For this review, take the finished solid that the model builds, in its own axes (mm). A direction names the side the tool comes from. Round coordinates to 2 decimals unless told otherwise and drop trailing zeros. Order: outer loops, then holes, each group sorted by start corner. A loop starts at its lowest first (then second) coordinate and runs counter-clockwise, first axis right, second up. Notation, with made-up numbers: (24.5, 24.5) - (74.5, 24.5) arc R30 ccw to (74.5, 46.5) - close; hole circle Ø11 at (89.5, -10). An arc over 180 degrees is marked (long way). One line per question, with ' | ' between items.
```python
from build123d import *

# Parameters (mm, degrees)
F1_DEPTH = 6.35


with BuildPart() as f1:
    # F0 (on Front) → F1 (new body)
    with BuildSketch(Plane.XZ):
        Polygon((-58.676012, 70.675433), (-59.716608, 71.344383), (-59.975654, 71.427517), (-59.975654, 71.006581), (-59.940577, 70.445329), (-59.71257, 70.129625), (-59.835345, 69.778845), (-59.800263, 69.357902), (-59.589796, 68.972044), (-59.168857, 68.410791), (-58.940846, 67.340903), (-58.432214, 66.691957), (-58.572527, 65.727308), (-58.917451, 65.727308), (-58.917451, 66.639341), (-58.917451, 67.017012), (-59.133779, 66.937506), (-59.965832, 69.201457), (-60.221203, 69.392987), (-60.431674, 69.11236), (-59.870422, 65.464221), (-59.291631, 64.341716), (-59.48456, 63.920781), (-60.690984, 62.307183), (-60.690984, 61.419144), (-60.169544, 60.334548), (-60.169544, 60.000826), (-59.794106, 59.416812), (-59.794106, 58.603365), (-59.522957, 57.93592), (-59.68982, 57.685629), (-59.251808, 56.767892), (-58.792941, 55.912729), (-59.126664, 54.911561), (-58.521792, 53.430669), (-58.792941, 53.15952), (-58.792941, 52.325215), (-58.462251, 51.65777), (-58.462251, 51.219761), (-58.462251, 43.550201), (-58.462251, 38.294077), (-57.80109, 22.979558), (-57.80109, 22.313071), (-57.328186, 18.700593), (-57.130594, 6.927098), (-56.944776, 2.058604), (-56.758955, -1.026015), (-56.944776, -5.597197), (-57.304534, -6.819496), (-57.532188, -12.329374), (-58.267996, -31.223956), (-58.635905, -31.775814), (-58.415901, -32.695577), (-58.415901, -36.606416), (-58.708549, -37.449244), (-58.708549, -37.89407), (-58.462724, -38.924195), (-58.462724, -47.071535), (-58.845624, -50.201591), (-59.208509, -56.475982), (-59.372392, -56.65157), (-59.372392, -57.037868), (-59.606511, -57.892401), (-59.442628, -58.255285), (-59.52654, -60.387559), (-59.52654, -64.487077), (-59.382007, -72.18682), (-57.002816, -72.18682), (-57.002816, -71.950309), (-57.002816, -68.186022), (-56.425326, -51.439133), (-55.987526, -46.775039), (-55.987526, -36.422912), (-55.72189, -28.219488), (-55.514717, -23.205277), (-55.412289, -19.943317), (-55.267755, -18.708207), (-55.267755, -18.497974), (-55.096943, -13.058227), (-54.540541, -5.07562), (-54.275367, -1.08695), (-54.39074, 1.474799), (-54.650679, 16.963238), (-54.650679, 24.818346), (-55.331245, 29.917276), (-55.331245, 34.031644), (-55.331245, 43.396994), (-55.628557, 43.991618), (-55.628557, 50.941303), (-55.628557, 52.09339), (-54.810949, 53.951591), (-55.10826, 55.103678), (-54.513637, 56.441586), (-53.956173, 57.370689), (-53.547371, 59.30322), (-54.253489, 60.715456), (-54.253489, 61.012767), (-54.253489, 62.350675), (-55.10826, 63.391268), (-55.10826, 64.023063), (-54.402143, 64.914994), (-55.294082, 67.404993), (-56.594826, 68.482749), (-57.635419, 69.374688), (-57.635419, 69.820657), align=None)
    extrude(amount=F1_DEPTH)


solid = f1.part
```
(1) For probe 1 along X at (y, z) = (-0.5, 61.5); probe 2 along X at (y, z) = (-1, -1), list the stretches that pass through material, from the lowest coordinate up. Write a range as [from, to].
Output values:
probe 1: [-60.69, -54.25] | probe 2: [-56.76, -54.28]
(2) We need section B-B on z = -62. State the section outline as (x, y) points.
Output values:
outline: (-59.53, -6.35) - (-56.79, -6.35) - (-56.79, 0) - (-59.53, 0) - close
(3) Mouldability with a two-part tool opening along Z and no side actions: class faces 1 (the flat face through (-54.986, -3.131, 27.332)), 2 (the flat face through (-56, -6.35, 1)), 3 (the flat face through (-54.41, -3.13, -3.11)) as released by +Z, released by -Z, zero draft, split by the parting line, or undercut.
Output values:
face 1: undercut | face 2: zero draft | face 3: released by -Z
(4) We need section A-A on z = -43.5. State the section outline as (x, y) points, plus the area to 3 significant figures.
Output values:
outline: (-58.46, -6.35) - (-55.99, -6.35) - (-55.99, 0) - (-58.46, 0) - close | area: 15.7 mm^2
(5) Insertion check: pin 1 (0.6 mm diameter, centred on y = -4.5, z = 66.5, fed in from +X); pin 2 (1 mm diameter, centred on y = -2, z = -25, fed in from +X); pin 3 (1.2 mm diameter, centred on y = -3.5, z = -34.5, fed in from -X). Each pin has a flat end and moves straight along its axis. Give the tip position at first contact, or say it passes through.
Output values:
pin 1: x = -54.86 | pin 2: x = -55.57 | pin 3: x = -58.42
(6) For faces 4 (the flat face through (-56.21, -3.13, -49.14)), 5 (the flat face through (-55.331, -3, 37)), 6 (the flat face through (-57.04, -3.13, 4.53)), list the 3-axis set-ups (+Z, -Z, +X, -X, +Y, -Y) from which the entire face can be reached by the end or side of a thin tool; tool diameter is ignored.
Output values:
face 4: -Z, +X, +Y, -Y | face 5: +X, +Y, -Y | face 6: -X, +Y, -Y
